Autodesk Inventor part; units mm, degrees
ref_plane "YZ Plane" through (0, 0, 0) normal (1, 0, 0) x (0, 1, 0)
ref_plane "XZ Plane" through (0, 0, 0) normal (0, 1, 0) x (-1, 0, 0)
ref_plane "XY Plane" through (0, 0, 0) normal (0, 0, 1) x (1, 0, 0)
sketch "Sketch1" plane through (0, 0, 0) normal (0, 0, 1) x (1, 0, 0)
  line L0 (0, 0) -> (-95.25, 0)
  line L1 (-95.25, 0) -> (-95.25, 66.675)
  line L2 (-95.25, 66.675) -> (0, 66.675)
  line L3 (0, 66.675) -> (0, 0)
  dimension "d0" = 66.675
  dimension "d1" = 95.25
extrude "Extrusion1" add sketch "Sketch1" along normal blind 3.175
sketch "Sketch2" plane through (0, 0, 3.175) normal (0, 0, 1) x (1, 0, 0)
  line L0 (-95.25, 0) -> (-95.25, 66.675)
  line L1 (0, 66.675) -> (0, 0)
  line L2 (-95.25, 66.675) -> (0, 66.675)
  line L3 (-95.25, 33.3375) -> (-95.25, 55.5625)
  line L4 (-47.625, 66.675) -> (-85.725, 66.675)
  line L5 (-85.725, 66.675) -> (-85.725, 55.5625)
  line L6 (-95.25, 33.3375) -> (-95.25, 11.1125)
  line L7 (-95.25, 11.1125) -> (-85.725, 11.1125)
  line L8 (-47.625, 66.675) -> (-9.525, 66.675)
  line L9 (-9.525, 66.675) -> (-9.525, 55.5625)
  line L10 (0, 11.1125) -> (-9.525, 11.1125)
  circle A0 centre (-85.725, 55.5625) radius 3.9687
  circle A1 centre (-9.525, 55.5625) radius 3.9688
  circle A2 centre (-85.725, 11.1125) radius 3.9688
  circle A3 centre (-9.525, 11.1125) radius 3.9688
  dimension "d4" = 22.225
  dimension "d5" = 38.1
  dimension "d6" = 22.225
  dimension "d7" = 38.1
  dimension "d8" = 7.9375
  dimension "d9" = 7.9375
  dimension "d10" = 7.9375
  dimension "d11" = 7.9375
extrude "Extrusion2" cut sketch "Sketch2" against normal blind 3.175
sketch "Sketch3" plane through (0, 0, 3.175) normal (0, 0, 1) x (1, 0, 0)
  circle A0 centre (-47.625, 33.3375) radius 6.35
  dimension "d14" = 12.7
extrude "Extrusion3" cut sketch "Sketch3" against normal blind 3.175
properties part number "mount plate"
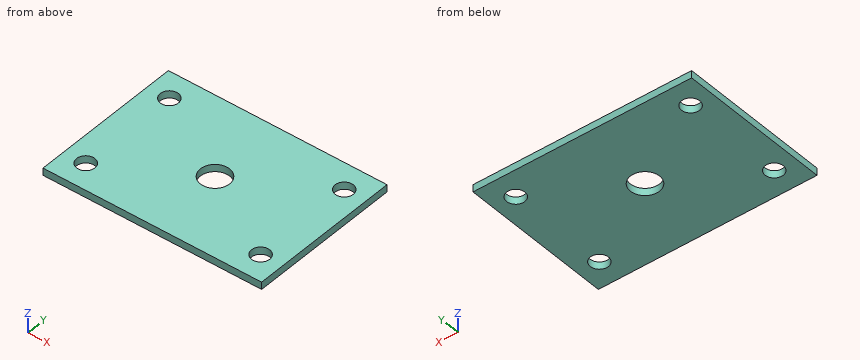
Verification items for the finished model (mm, model axes). Coordinates: 2 decimals unless noted, no trailing zeros. Order: outer loops, then holes, each group sorted by start corner. A loop starts at its lowest first (then second) coordinate and runs counter-clockwise, first axis right, second up. Notation, with made-up numbers: (56, 26.5) -> (96, 26.5) arc R20 ccw to (96, 33.5) -> close; hole circle Ø7 at (23.5, 25). An arc over 180 degrees is marked (long way). Answer as CSV lines item,"result". Start each with the question number.
1) Material ranges on L1, parallel to X at y = 10, z = 2.85; L2, parallel to X at y = 33.5, z = 0.75; L3, parallel to X at y = 8, z = 0.2, recorded low to high. Write a range as [from, to].
2) Cross-section at A-A, the plane y = 58. Record the boundary of the cut face in (x, z) (3 decimals), then the cut area to 3 significant figures.
3) Cross-section at D-D, the plane y = 28.5. Record the boundary of the cut face in (x, z) (3 decimals), then the cut area to 3 significant figures.
4) Gauge pin test, flat end, axial feed: pin 1 Ø7 at (x, y) = (-9.52, 11.11) entering from -Z. Record the tip position at first contact, or that the pin passes through.
5) Cross-section at B-B, the plane x = -51. Record the boundary of the cut face in (y, z) (3 decimals), then the cut area to 3 significant figures.
6) Cross-section at C-C, the plane z = 1.25. Give the number of separate pieces and of enclosed holes in the cut face, then the cut area to 3 significant figures.
Conclusion:
1,L1,"x = [-95.25, -89.53], [-81.92, -13.33], [-5.72, 0]"
1,L2,"x = [-95.25, -53.97], [-41.28, 0]"
1,L3,"x = [-95.25, -88.19], [-83.26, -11.99], [-7.06, 0]"
2,outline,"(-95.25, 0) -> (-88.857, 0) -> (-88.857, 3.175) -> (-95.25, 3.175) -> close; (-82.593, 0) -> (-12.657, 0) -> (-12.657, 3.175) -> (-82.593, 3.175) -> close; (-6.393, 0) -> (0, 0) -> (0, 3.175) -> (-6.393, 3.175) -> close"
2,area,"263 mm²"
3,outline,"(-95.25, 0) -> (-51.739, 0) -> (-51.739, 3.175) -> (-95.25, 3.175) -> close; (-43.511, 0) -> (0, 0) -> (0, 3.175) -> (-43.511, 3.175) -> close"
3,area,"276 mm²"
4,pin 1,"passes through"
5,outline,"(0, 0) -> (27.959, 0) -> (27.959, 3.175) -> (0, 3.175) -> close; (38.716, 0) -> (66.675, 0) -> (66.675, 3.175) -> (38.716, 3.175) -> close"
5,area,"178 mm²"
6,separate pieces,"1"
6,enclosed holes,"5"
6,area,"6,030 mm²"
